The model under review builds one solid part; all positions refer to its coordinate system, in mm. Round coordinates to 2 decimals unless told otherwise and drop trailing zeros. Loops run counter-clockwise (first coordinate to the right, second up) from the corner with the lowest first, then second, coordinate; pieces in that order, holes last. Notation, with made-up numbers: (66, -11.5) -> (83, -11.5) arc R24 ccw to (83, 15.5) -> close; hole circle Ø6 at (-6, -35.5). An arc over 180 degrees is marked (long way). Use a Markdown table: item, result. Add a question column.
1) Insertion check: pin 1 (5 mm diameter, centred on x = 152, y = 106.5, fed in from +Z); pin 2 (0.5 mm diameter, centred on x = -9.5, z = 3.5, fed in from +Y); pin 3 (4 mm diameter, centred on x = 11.5, y = 79, fed in from +Z). Each pin has a flat end and moves straight along its axis. Give the tip position at first contact, or say it passes through.
2) Mouldability with a two-part tool opening along X and no side actions: class faces 1 (the flat face through (-2, 1, 2.8)), 2 (the flat face through (-3, -4, 0)) as released by +X, released by -X, zero draft, split by the parting line, or undercut.
3) Consider section C-C on y = -20. Give the boundary of the cut face in (x, z).
4) Consider section B-B on z = 1.75. Give the boundary of the cut face in (x, y).
5) Wall thickness on probe 1 along X at (y, z) = (106.6, 0.95); probe 2 along Y at (x, z) = (-156.5, 0.95); probe 3 along Y at (x, z) = (83, 3.2): over which ranges is each line inside the solid? List them lowest first.
6) Consider section A-A on x = -94. Give the boundary of the cut face in (y, z).
from build123d import *

# Parameters (mm, degrees)
F0_W      = 360
F0_H      = 207
F1_DEPTH  = 3.8
F2_R      = 5
F3_W      = 349.1
F3_H      = 198
F4_DEPTH  = 1
F6_W      = 13
F6_H      = 6.3
F6_W_2    = 15
F7_DEPTH  = 0.3
F8_R      = 2.4
F9_R      = 1.2
F10_DEPTH = 1.101
F11_W     = 251
F11_H     = 10.5
F12_DEPTH = 3.8


with BuildPart() as f1:
    # F0 (on Top) → F1 (new body)
    with BuildSketch(Plane.XY):
        Rectangle(F0_W, F0_H)
    extrude(amount=F1_DEPTH)

    # F2
    f2_edges = [f1.edges().sort_by_distance(p)[0] for p in [
        (180, 103.5, 1.9),
        (-180, 103.5, 1.9),
        (-180, -103.5, 1.9),
        (180, -103.5, 1.9),
    ]]
    fillet(f2_edges, radius=F2_R)

    # F3 (on face) → F4 (cut)
    with BuildSketch(Plane.XY.offset(3.8)):
        Rectangle(F3_W, F3_H)
    extrude(amount=-F4_DEPTH, mode=Mode.SUBTRACT)

    # F6 (on offset) → F7 (join)
    with BuildSketch(Plane.XY.offset(0.8)):
        with Locations((-153.5, 106.65)):
            Rectangle(F6_W, F6_H)
        with Locations((153.5, 106.65)):
            Rectangle(F6_W, F6_H)
        with Locations((-152.5, -106.65)):
            Rectangle(F6_W_2, F6_H)
        with Locations((152.5, -106.65)):
            Rectangle(F6_W_2, F6_H)
    extrude(amount=F7_DEPTH)

    # F8
    f8_edges = [f1.edges().sort_by_distance(p)[0] for p in [
        (-160, 109.8, 0.95),
        (-147, 109.8, 0.95),
        (147, 109.8, 0.95),
        (160, 109.8, 0.95),
        (145, -109.8, 0.95),
        (160, -109.8, 0.95),
        (-160, -109.8, 0.95),
        (-145, -109.8, 0.95),
    ]]
    fillet(f8_edges, radius=F8_R)

    # F9 (on face) → F10 (cut, through all)
    with BuildSketch(Plane.XY.offset(1.1)):
        with Locations((-156.5, 106.6)):
            Circle(F9_R)
        with Locations((-150.5, 106.6)):
            Circle(F9_R)
        with Locations((150.5, 106.6)):
            Circle(F9_R)
        with Locations((156.5, 106.6)):
            Circle(F9_R)
        with Locations((148.5, -106.7)):
            Circle(F9_R)
        with Locations((156.5, -106.7)):
            Circle(F9_R)
        with Locations((-156.5, -106.7)):
            Circle(F9_R)
        with Locations((-148.5, -106.7)):
            Circle(F9_R)
    extrude(amount=-F10_DEPTH, mode=Mode.SUBTRACT)

    # F11 (on Top) → F12 (join)
    with BuildSketch(Plane.XY):
        with Locations((0, -108.75)):
            Rectangle(F11_W, F11_H)
    extrude(amount=F12_DEPTH)


solid = f1.part
Result set:
| question | item | result |
|---|---|---|
| 1 | pin 1 | z = 1.1 |
| 1 | pin 2 | y = 103.5 |
| 1 | pin 3 | z = 2.8 |
| 2 | face 1 | undercut |
| 2 | face 2 | zero draft |
| 3 | outline | (-180, 0) -> (180, 0) -> (180, 3.8) -> (174.55, 3.8) -> (174.55, 2.8) -> (-174.55, 2.8) -> (-174.55, 3.8) -> (-180, 3.8) -> close |
| 4 | outline | (-180, -98.5) arc R5 ccw to (-175, -103.5) -> (-125.5, -103.5) -> (-125.5, -114) -> (125.5, -114) -> (125.5, -103.5) -> (175, -103.5) arc R5 ccw to (180, -98.5) -> (180, 98.5) arc R5 ccw to (175, 103.5) -> (-175, 103.5) arc R5 ccw to (-180, 98.5) -> close |
| 5 | probe 1 | -160 to -157.7, -155.3 to -151.7, -149.3 to -147, 147 to 149.3, 151.7 to 155.3, 157.7 to 160 |
| 5 | probe 2 | -109.8 to -107.9, -105.5 to 105.4, 107.8 to 109.8 |
| 5 | probe 3 | -114 to -99, 99 to 103.5 |
| 6 | outline | (-114, 0) -> (103.5, 0) -> (103.5, 3.8) -> (99, 3.8) -> (99, 2.8) -> (-99, 2.8) -> (-99, 3.8) -> (-114, 3.8) -> close |
